Work out the finished part from the listing and answer in its coordinate system (mm). A direction names the side the tool comes from. Coordinates: 2 decimals unless noted, no trailing zeros. Order: outer loops, then holes, each group sorted by start corner. A loop starts at its lowest first (then second) coordinate and runs counter-clockwise, first axis right, second up.
Autodesk Inventor part; units mm, degrees
ref_plane "YZ Plane" through (0, 0, 0) normal (1, 0, 0) x (0, 1, 0)
ref_plane "XZ Plane" through (0, 0, 0) normal (0, 1, 0) x (-1, 0, 0)
ref_plane "XY Plane" through (0, 0, 0) normal (0, 0, 1) x (1, 0, 0)
sketch "スケッチ1" plane through (0, 0, 0) normal (0, 0, 1) x (1, 0, 0)
  circle A0 centre (0, 0) radius 10.35
  circle A1 centre (0, 0) radius 3.2
  dimension "d0" = 20.7
  dimension "d1" = 6.4
extrude "押し出し1" add sketch "スケッチ1" along normal blind 110
sketch "スケッチ2" plane through (0, 0, 0) normal (0, 0, -1) x (-1, 0, 0)
  circle A0 centre (0, 0) radius 3.2
  circle A1 centre (0, 0) radius 5.5
  dimension "d4" = 11
extrude "押し出し2" add sketch "スケッチ2" along normal blind 20
fillet "フィレット1" radius 6 1 edges at (5.5, 0, 0)
properties part number "gpu_supporter_01"
1. For faces 1 (the cylindrical face through (1.19, 5.37, -12.85)), 2 (the flat face through (-2.4, 2.4, 110)), determine the directions among +Z, -Z, +X, -X, +Y, -Y from which every point of the face is accessible in a straight line to the end or side of a thin tool.
2. Flat-ended cylindrical pins translate along their axes: pin 1 (2 mm diameter, centred on x = 5, z = 39.5, fed in from -Y); pin 2 (8 mm diameter, centred on x = -4, z = 26.5, fed in from -Y); pin 3 (4 mm diameter, centred on x = -4.5, z = 77.5, fed in from -Y); pin 4 (1.5 mm diameter, centred on y = 4.5, z = 86.5, fed in from +X). Find the tip coordinate at first contact, or state that the pin passes through.
3. The part is cut by section A-A (y = 0). Determine the outline of the cut face in (x, z), plus the area to 3 significant figures.
4. Consider probe 1 along X at (y, z) = (0, -5.5); probe 2 along Y at (x, z) = (0, -7); probe 3 along X at (y, z) = (0, 71.5). Determine where each line is inside the solid, lowest interval first.
5. The part is cut by section C-C (z = -7.5). Determine the outline of the cut face in (x, y).
Worked out:
1. face 1: -Z
1. face 2: +Z, +X, -X, +Y, -Y
2. pin 1: stops at y = -9.55
2. pin 2: stops at y = -10.35
2. pin 3: stops at y = -10.04
2. pin 4: stops at x = 9.65
3. outline: (-10.35, 0) arc R6 cw to (-5.5, -5.89) - (-5.5, -20) - (-3.2, -20) - (-3.2, 110) - (-10.35, 110) - close; (3.2, -20) - (5.5, -20) - (5.5, -5.89) arc R6 cw to (10.35, 0) - (10.35, 110) - (3.2, 110) - close
3. area: 1,680 mm2
4. probe 1: x = -5.51 to -3.2, 3.2 to 5.51
4. probe 2: y = -5.5 to -3.2, 3.2 to 5.5
4. probe 3: x = -10.35 to -3.2, 3.2 to 10.35
5. outline: circle Ø11 at (0, 0); hole circle Ø6.4 at (0, 0)
